Check sheet for the modelled part. Datum: model origin and axes. Units: mm. A direction names the side the tool comes from. Round coordinates to 2 decimals unless told otherwise and drop trailing zeros. Loops run counter-clockwise (first coordinate to the right, second up) from the corner with the lowest first, then second, coordinate; pieces in that order, holes last. Notation, with made-up numbers: (73, -10) -> (84, -10) arc R32 ccw to (84, 18) -> close; hole circle Ø4 at (21, 25). An arc over 180 degrees is marked (long way). Use one line per item in the form item = value. Start each with the question number.
(1) Go/stop test with flat-tipped pins: pin 1 (4.5 mm diameter, centred on y = -4.5, z = 7, fed in from +X); pin 2 (4.5 mm diameter, centred on x = 22.5, z = 10, fed in from -Y); pin 3 (2 mm diameter, centred on x = 135.5, z = 8.5, fed in from -Y). Record where each tip stops, or that it passes through.
(2) Material ranges on probe 1 along X at (y, z) = (14.5, 9.5); probe 2 along X at (y, z) = (11, 2); probe 3 along Y at (x, z) = (-17, 6), recorded low to high. Write a range as [from, to].
(3) Sectioned sample at A-A (y = 12). Record the cut outline in (x, z), and give its area (3 significant figures).
(4) Draft check along X on faces 1 (the flat face through (78, 25, 0)), 2 (the flat face through (-33, 0.999, 7)), 3 (the flat face through (-56.627, 14, 7)). Enter one of: released by +X, released by -X, zero draft, split by the parting line, or undercut.
(5) Sectioned sample at C-C (y = -3). Record the cut outline in (x, z), and give its area (3 significant figures).
(6) Sectioned sample at B-B (z = 2.75). Record the cut outline in (x, y), and give its area (3 significant figures).
(7) Set-up check for faces 4 (the flat face through (78, 25, 15)), 5 (the flat face through (-36.627, 8, 7)), 6 (the flat face through (22, 40.999, 7)): record each of +Z, -Z, +X, -X, +Y, -Y from which the full face is reachable in a straight line by a thin tool's end or side.
(8) Sectioned sample at D-D (x = -18). Record the cut outline in (y, z), and give its area (3 significant figures).
from build123d import *

# Parameters (mm, degrees)
F0_R     = 17.5
F0_W     = 10
F0_H     = 30
F0_W_2   = 8
F0_H_2   = 15
F1_DEPTH = 15


with BuildPart() as f1:
    # F0 (on Top) → F1 (new body)
    with BuildSketch(Plane.XY):
        Polygon((98.3732019503, 40.9987986088), (-56.6267980497, 40.9987986088), (-56.6267980497, 15.9987986088), (-46.6267980497, 15.9987986088), (-36.6267980497, 15.9987986088), (-28.6267980497, 15.9987986088), (-18.6267980497, 15.9987986088), (-11.6267980497, 15.9987986088), (-4.6267980497, 15.9987986088), (98.3732019503, 15.9987986088), align=None)
        with BuildLine():
            ThreePointArc((98.3732019503, 15.9987986088), (166.0649440268, 28.4987986088), (98.3732019503, 40.9987986088))
            Line((98.3732019503, 40.9987986088), (98.3732019503, 15.9987986088))
        make_face()
        with Locations((131.0649440268, 28.4987986088)):
            Circle(F0_R, mode=Mode.SUBTRACT)
        with Locations((131.0649440268, 28.4987986088)):
            Circle(F0_R)
        with Locations((-51.6267980497, 0.9987986088)):
            Rectangle(F0_W, F0_H)
        with Locations((-32.6267980497, 8.4987986088)):
            Rectangle(F0_W_2, F0_H_2)
    extrude(amount=F1_DEPTH)


solid = f1.part
Checks:
q1.pin_1 = 147.78
q1.pin_2 = 16
q1.pin_3 = -6.33
q2.probe_1 = [-56.63, -46.63], [-36.63, -28.63], [98.99, 163.14]
q2.probe_2 = [-56.63, -46.63], [-36.63, -28.63], [100.75, 161.38]
q2.probe_3 = [16, 41]
q3.outline = (-56.63, 0) -> (-46.63, 0) -> (-46.63, 15) -> (-56.63, 15) -> close; (-36.63, 0) -> (-28.63, 0) -> (-28.63, 15) -> (-36.63, 15) -> close; (100.2, 0) -> (161.93, 0) -> (161.93, 15) -> (100.2, 15) -> close
q3.area = 1,200 mm2
q4.face_1 = zero draft
q4.face_2 = undercut
q4.face_3 = released by -X
q5.outline = (-56.63, 0) -> (-46.63, 0) -> (-46.63, 15) -> (-56.63, 15) -> close; (115.81, 0) -> (146.32, 0) -> (146.32, 15) -> (115.81, 15) -> close
q5.area = 608 mm2
q6.outline = (-56.63, -14) -> (-46.63, -14) -> (-46.63, 16) -> (-36.63, 16) -> (-36.63, 1) -> (-28.63, 1) -> (-28.63, 16) -> (98.37, 16) arc R35 ccw (long way) to (98.37, 41) -> (-56.63, 41) -> close
q6.area = 8,100 mm2
q7.face_4 = +Z, +X, -X, +Y, -Y
q7.face_5 = +Z, -Z, -Y
q7.face_6 = +Z, -Z, -X, +Y
q8.outline = (16, 0) -> (41, 0) -> (41, 15) -> (16, 15) -> close
q8.area = 375 mm2
